Input: dimensioned drawing with shaded views. Units: mm. Origin: part minimum x, y, z. A direction names the side the tool comes from. Coordinates: 2 decimals unless noted, no trailing zeros. Order: outer loops, then holes, each group sorted by start corner. A loop starts at its lowest first (then second) coordinate and runs counter-clockwise, first axis right, second up. Notation, with made-up numbers: (81, 47) -> (102, 47) arc R25 cw to (102, 83) -> close; hole circle Ø11 at (82.25, -38). An arc over 180 degrees is marked (long way). Answer in a Markdown table with one row per item. Add a question column.
1) Section query D-D on y = 35.7. Return the cut outline in (x, z), then the cut area to 3 significant figures.
2) Contact query for flat-ended pins moving along their axis: P1, Ø1.5, axis at x = 35, y = 20, coming from the +Z side; P2, Ø6, axis at y = 22.5, z = 12.5, coming from the +X side. Output: stop coordinate, or through.
3) Section query B-B on z = 10.5. Return the cut outline in (x, y).
4) Section query A-A on z = 5. Return the cut outline in (x, y), then the cut area to 3 significant figures.
5) Set-up query: the marked faces 1 and 2. Return all of +Z, -Z, +X, -X, +Y, -Y with unobstructed straight access to the full face (end or side cutting, diameter ignored); none if empty.
6) Section query C-C on x = 31.5. Return the cut outline in (y, z), then the cut area to 4 significant figures.
7) Pull-direction query (Y, two-part tool) for the marked faces 3, 4 and 5; classes: +Y half, -Y half, draft (parallel to the pull), parting line (faces both ways), or undercut.
8) Ray query, line 1 (X direction, y = 26, z = 7.75); line 2 (Y direction, x = 20, z = 4); line 3 (Z direction, x = 22.5, y = 8.5). Return the intervals inside material, ascending. Write a range as from..to.
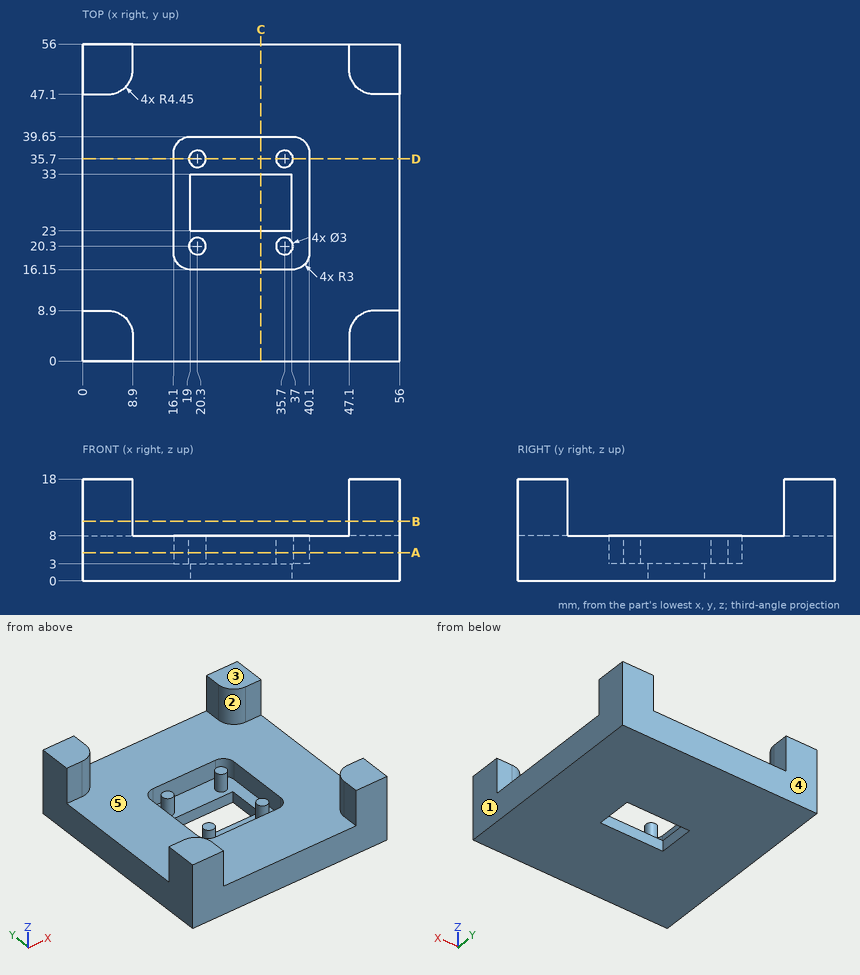
Result:
| question | item | result |
|---|---|---|
| 1 | outline | (0, 0) -> (56, 0) -> (56, 8) -> (40.1, 8) -> (40.1, 3) -> (37.2, 3) -> (37.2, 8) -> (34.2, 8) -> (34.2, 3) -> (21.8, 3) -> (21.8, 8) -> (18.8, 8) -> (18.8, 3) -> (16.1, 3) -> (16.1, 8) -> (0, 8) -> close |
| 1 | area | 358 mm2 |
| 2 | P1 | z = 8 |
| 2 | P2 | through |
| 3 | outline | (0, 0) -> (8.9, 0) -> (8.9, 4.45) arc R4.45 ccw to (4.45, 8.9) -> (0, 8.9) -> close; (0, 47.1) -> (4.45, 47.1) arc R4.45 ccw to (8.9, 51.55) -> (8.9, 56) -> (0, 56) -> close; (47.1, 0) -> (56, 0) -> (56, 8.9) -> (51.55, 8.9) arc R4.45 ccw to (47.1, 4.45) -> close; (47.1, 51.55) arc R4.45 ccw to (51.55, 47.1) -> (56, 47.1) -> (56, 56) -> (47.1, 56) -> close |
| 4 | outline | (0, 0) -> (56, 0) -> (56, 56) -> (0, 56) -> close; circle Ø3 at (20.3, 20.3); circle Ø3 at (20.3, 35.7); circle Ø3 at (35.7, 20.3); circle Ø3 at (35.7, 35.7); hole (16.1, 19.15) arc R3 ccw to (19.1, 16.15) -> (37.1, 16.15) arc R3 ccw to (40.1, 19.15) -> (40.1, 36.65) arc R3 ccw to (37.1, 39.65) -> (19.1, 39.65) arc R3 ccw to (16.1, 36.65) -> close |
| 4 | area | 2,610 mm2 |
| 5 | face 1 | +Z, -Z, +X, +Y, -Y |
| 5 | face 2 | +Z |
| 6 | outline | (0, 0) -> (23, 0) -> (23, 3) -> (16.15, 3) -> (16.15, 8) -> (0, 8) -> close; (33, 0) -> (56, 0) -> (56, 8) -> (39.65, 8) -> (39.65, 3) -> (33, 3) -> close |
| 6 | area | 300.5 mm2 |
| 7 | face 3 | draft |
| 7 | face 4 | +Y half |
| 7 | face 5 | undercut |
| 8 | line 1 | 0..16.1, 40.1..56 |
| 8 | line 2 | 0..16.15, 18.83..21.77, 34.23..37.17, 39.65..56 |
| 8 | line 3 | 0..8 |
